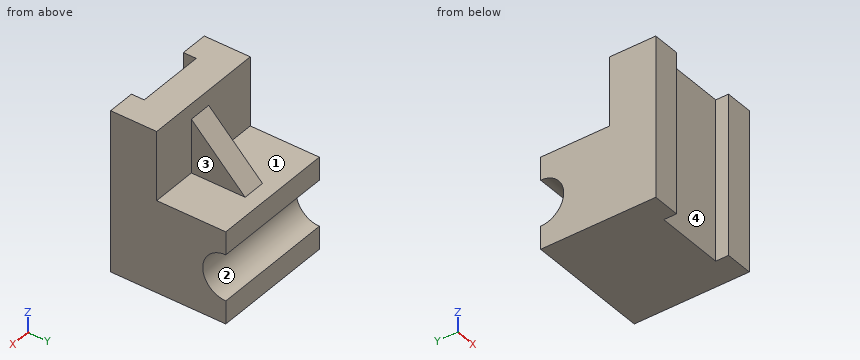
```python
from build123d import *

# Parameters (mm, degrees)
BOSS_EXTRUDE1_DEPTH = 54
SKETCH2_R           = 10
CUT_EXTRUDE1_DEPTH  = 84.555784218
RIB4_REACH          = 74.26
SKETCH5_WALL_W      = 188.871183906
SKETCH5_WALL_H      = 10
SKETCH6_W           = 30
SKETCH6_H           = 11.131491479
CUT_EXTRUDE2_DEPTH  = 101.562854881


with BuildPart() as part:
    # Sketch1 → Boss-Extrude1 (new body)
    with BuildSketch(Plane(origin=(0, 0, 0), x_dir=(0, 0, -1), z_dir=(1, 0, 0))):
        Polygon((42.055692771, 47.925857131), (2.055692771, 47.925857131), (2.055692771, 17.925857131), (-27.944307229, 17.925857131), (-27.944307229, -2.074142869), (42.055692771, -2.074142869), align=None)
    extrude(amount=BOSS_EXTRUDE1_DEPTH)

    # Sketch2 → Cut-Extrude1 (cut, through all)
    with BuildSketch(Plane(origin=(54, 0, 0), x_dir=(0, 0, -1), z_dir=(1, 0, 0))):
        with Locations((22.055692771, 47.925857131)):
            Circle(SKETCH2_R)
    extrude(amount=-CUT_EXTRUDE1_DEPTH, mode=Mode.SUBTRACT)

    # Sketch5 wall → Rib4 (add, up to next)
    with BuildSketch(Plane(origin=(34, 28.80129121, 10.41851211), x_dir=(0, -0.707106781187, 0.707106781187), z_dir=(0, -0.707106781187, -0.707106781187)), mode=Mode.PRIVATE) as rib4_sk1:
        with Locations((0, 5)):
            Rectangle(SKETCH5_WALL_W, SKETCH5_WALL_H)
    rib4_tool1 = extrude(rib4_sk1.sketch, amount=RIB4_REACH, mode=Mode.PRIVATE) - part.part
    add(rib4_tool1.solids().sort_by_distance((34, 28.80129121, 10.41851211))[0])

    # Sketch6 → Cut-Extrude2 (cut, through all)
    with BuildSketch(Plane.XY.offset(27.944307229)):
        with Locations((27, -2.074142869)):
            Rectangle(SKETCH6_W, SKETCH6_H)
    extrude(amount=-CUT_EXTRUDE2_DEPTH, mode=Mode.SUBTRACT)


solid = part.part
```
Input: part model. Units: mm. Frame: model coordinates. Face numbers are marked on the shaded views. A direction names the side the tool comes from. Coordinates: 2 decimals unless noted, no trailing zeros. Write each loop counter-clockwise with the first axis right and the second up, starting at its lowest first coordinate (ties: lowest second). Pieces come first, ordered by that corner, then holes. Notation, with made-up numbers: (9.5, 67) - (34.5, 67) arc R21 cw to (34.5, 96) - close; hole circle Ø11 at (-17.5, 2). An arc over 180 degrees is marked (long way). Put each result on its own line as item: value. Start each with the question number.
1) Cut plane B-B (z = 23.5). Return the cut outline in (x, y).
2) Cut plane C-C (z = 16). Return the cut outline in (x, y).
3) Contact query for flat-ended pins moving along their axis: pin 1 (8 mm diameter, centred on x = 18, y = 34.5, fed in from +Z); pin 2 (15 mm diameter, centred on x = 26.5, z = -11.5, fed in from -Y); pin 3 (11.5 mm diameter, centred on y = 24.5, z = 14, fed in from -X). Output: stop coordinate, or through.
4) Ray query, L1, parallel to X at y = 2, z = -28; L2, parallel to Y at x = 17, z = 10; L3, parallel to Y at x = 4.5, z = -1.5. Return the intervals inside material, ascending.
5) Cut plane A-A (x = 23). Return the cut outline in (y, z), plus the area to 3 significant figures.
6) Reachability of the marked faces 1, 2, 3 and 4 from +Z, -Z, +X, -X, +Y, -Y: full face, straight path, thin tool, end or side. Return the list, or none.
Resolved:
1. outline: (0, -2.07) - (12, -2.07) - (12, 3.49) - (42, 3.49) - (42, -2.07) - (54, -2.07) - (54, 17.93) - (0, 17.93) - close
2. outline: (0, -2.07) - (12, -2.07) - (12, 3.49) - (42, 3.49) - (42, -2.07) - (54, -2.07) - (54, 17.93) - (34, 17.93) - (34, 23.22) - (24, 23.22) - (24, 17.93) - (0, 17.93) - close
3. pin 1: stops at z = -2.06
3. pin 2: stops at y = 3.49
3. pin 3: stops at x = 24
4. L1: x = 0 to 12, 42 to 54
4. L2: y = 3.49 to 17.93
4. L3: y = -2.07 to 17.93
5. outline: (3.49, -42.06) - (47.93, -42.06) - (47.93, -32.06) arc R10 cw to (47.93, -12.06) - (47.93, -2.06) - (17.93, -2.06) - (17.93, 27.94) - (3.49, 27.94) - close
5. area: 2,050 mm2
6. face 1: +Z, +Y
6. face 2: +X, -X, +Y
6. face 3: +Z, +X, +Y
6. face 4: +Z, -Z, -Y
